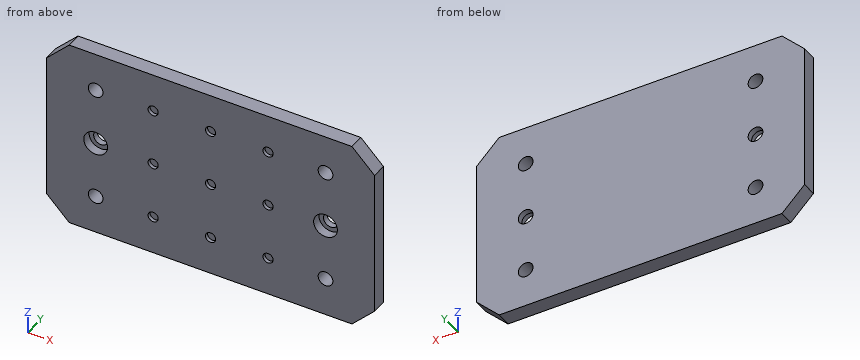
from build123d import *

# Parameters (mm, degrees)
SKETCH1_W           = 145
SKETCH1_H           = 85
BOSS_EXTRUDE1_DEPTH = 6.6
SKETCH2_R           = 3.25
CUT_EXTRUDE1_DEPTH  = 85.297449546
CHAMFER1_SIZE       = 10
CUT_EXTRUDE2_START  = -4
SKETCH3_R           = 5.25
SKETCH3_R_2         = 3.25
CUT_EXTRUDE2_DEPTH  = 4
SKETCH4_R           = 2.25
CUT_EXTRUDE3_DEPTH  = 1.5


with BuildPart() as part:
    # Sketch1 → Boss-Extrude1 (new body)
    with BuildSketch(Plane(origin=(0, 0, 0), x_dir=(1, 0, 0), z_dir=(0, 1, 0))):
        Rectangle(SKETCH1_W, SKETCH1_H)
    extrude(amount=BOSS_EXTRUDE1_DEPTH)

    # Sketch2 → Cut-Extrude1 (cut, through all)
    with BuildSketch(Plane(origin=(0, 6.6, 0), x_dir=(1, 0, 0), z_dir=(0, 1, 0))):
        with Locations(Location((-50.8, 25.4, 0), (0, 0, 270))):
            Circle(SKETCH2_R)
        with Locations(Location((50.8, 25.4, 0), (0, 0, 270))):
            Circle(SKETCH2_R)
        with Locations(Location((50.8, -25.4, 0), (0, 0, 270))):
            Circle(SKETCH2_R)
        with Locations(Location((-50.8, -25.4, 0), (0, 0, 270))):
            Circle(SKETCH2_R)
        with Locations(Location((50.8, 0, 0), (0, 0, 270))):
            Circle(SKETCH2_R)
        with Locations(Location((-50.8, 0, 0), (0, 0, 90))):
            Circle(SKETCH2_R)
    extrude(amount=-CUT_EXTRUDE1_DEPTH, mode=Mode.SUBTRACT)

    # Chamfer1
    chamfer1_edges = [part.edges().sort_by_distance(p)[0] for p in [
        (72.5, 3.3, 42.5),
        (-72.5, 3.3, 42.5),
        (-72.5, 3.3, -42.5),
        (72.5, 3.3, -42.5),
    ]]
    chamfer(chamfer1_edges, length=CHAMFER1_SIZE)

    # Sketch3 → Cut-Extrude2 (cut)
    # profile 1 of 2: a face of its own
    with BuildSketch(Plane.XZ.offset(CUT_EXTRUDE2_START)):
        with Locations(Location((50.8, 0, 0), (0, 0, 270))):
            Circle(SKETCH3_R)
        with Locations(Location((50.8, 0, 0), (0, 0, 90))):
            Circle(SKETCH3_R_2, mode=Mode.SUBTRACT)
    # profile 2 of 2: a face of its own
    with BuildSketch(Plane.XZ.offset(CUT_EXTRUDE2_START)):
        with Locations(Location((-50.8, 0, 0), (0, 0, 270))):
            Circle(SKETCH3_R)
        with Locations(Location((-50.8, 0, 0), (0, 0, 270))):
            Circle(SKETCH3_R_2, mode=Mode.SUBTRACT)
    extrude(amount=CUT_EXTRUDE2_DEPTH, mode=Mode.SUBTRACT)

    # Sketch4 → Cut-Extrude3 (cut)
    with BuildSketch(Plane.XZ):
        with Locations(Location((-25.4, 25.4, 0), (0, 0, 270))):
            Circle(SKETCH4_R)
        with Locations(Location((0, 25.4, 0), (0, 0, 270))):
            Circle(SKETCH4_R)
        with Locations(Location((25.4, 25.4, 0), (0, 0, 270))):
            Circle(SKETCH4_R)
        with Locations(Location((-25.4, 0, 0), (0, 0, 270))):
            Circle(SKETCH4_R)
        with Locations(Location((0, 0, 0), (0, 0, 270))):
            Circle(SKETCH4_R)
        with Locations(Location((25.4, 0, 0), (0, 0, 270))):
            Circle(SKETCH4_R)
        with Locations(Location((-25.4, -25.4, 0), (0, 0, 270))):
            Circle(SKETCH4_R)
        with Locations(Location((0, -25.4, 0), (0, 0, 270))):
            Circle(SKETCH4_R)
        with Locations(Location((25.4, -25.4, 0), (0, 0, 270))):
            Circle(SKETCH4_R)
    extrude(amount=-CUT_EXTRUDE3_DEPTH, mode=Mode.SUBTRACT)


solid = part.part
Part model, mm, in its own coordinate system. Round coordinates to 2 decimals unless told otherwise and drop trailing zeros. Loops run counter-clockwise (first coordinate to the right, second up) from the corner with the lowest first, then second, coordinate; pieces in that order, holes last. Notation, with made-up numbers: (32.25, 3.25) - (40.25, 3.25) arc R20 ccw to (40.25, 20.25) - close; hole circle Ø7 at (61.25, 82.5). An arc over 180 degrees is marked (long way). Answer as a JSON object with one key per item and string values.
Item 1: Band-saw the part on D-D on x = 25.4. List the corners of the cut face in (y, z).
Output:
{"outline": "(0, -42.5) - (6.6, -42.5) - (6.6, 42.5) - (0, 42.5) - (0, 27.65) - (1.5, 27.65) - (1.5, 23.15) - (0, 23.15) - (0, 2.25) - (1.5, 2.25) - (1.5, -2.25) - (0, -2.25) - (0, -23.15) - (1.5, -23.15) - (1.5, -27.65) - (0, -27.65) - close"}
Item 2: Wall check: L1, parallel to X at y = 1.75, z = 25.4; L2, parallel to X at y = 3.75, z = -4; L3, parallel to Z at x = -55.5, y = 2. Give the ranges that are in metal, low to high.
Output:
{"L1": "-72.5 to -54.05, -47.55 to 47.55, 54.05 to 72.5", "L2": "-72.5 to -54.2, -47.4 to 47.4, 54.2 to 72.5", "L3": "-42.5 to -2.34, 2.34 to 42.5"}
Item 3: Band-saw the part on A-A on x = 50.8. List the corners of the cut face in (y, z).
Output:
{"outline": "(0, -42.5) - (6.6, -42.5) - (6.6, -28.65) - (0, -28.65) - close; (0, -22.15) - (6.6, -22.15) - (6.6, -3.25) - (4, -3.25) - (4, -5.25) - (0, -5.25) - close; (0, 5.25) - (4, 5.25) - (4, 3.25) - (6.6, 3.25) - (6.6, 22.15) - (0, 22.15) - close; (0, 28.65) - (6.6, 28.65) - (6.6, 42.5) - (0, 42.5) - close"}
Item 4: Band-saw the part on C-C on y = 5.5. List the corners of the cut face in (x, z).
Output:
{"outline": "(-72.5, -32.5) - (-62.5, -42.5) - (62.5, -42.5) - (72.5, -32.5) - (72.5, 32.5) - (62.5, 42.5) - (-62.5, 42.5) - (-72.5, 32.5) - close; hole circle Ø6.5 at (-50.8, -25.4); hole circle Ø6.5 at (-50.8, 0); hole circle Ø6.5 at (-50.8, 25.4); hole circle Ø6.5 at (50.8, -25.4); hole circle Ø6.5 at (50.8, 0); hole circle Ø6.5 at (50.8, 25.4)"}
Item 5: Pin check, flat tips, straight feed: pin 1 (2 mm diameter, centred on x = 25, z = 26.5, fed in from -Y); pin 2 (9.5 mm diameter, centred on x = -50.8, z = 0, fed in from -Y); pin 3 (6 mm diameter, centred on x = 50.8, z = 25.4, fed in from +Y). Stop position of each tip, or through.
Output:
{"pin 1": "y = 1.5", "pin 2": "y = 4", "pin 3": "through"}
Item 6: Band-saw the part on B-B on z = 0. State how many separate pieces and enclosed holes the cut face has, plus the area to 3 significant figures.
Output:
{"separate pieces": "3", "enclosed holes": "0", "area": "819 mm2"}
